from build123d import *

# Parameters (mm, degrees)
SKETCH_1_W          = 95
SKETCH_1_H          = 36
SKETCH_1_R          = 1.75
EXTRUDE_1_DEPTH     = 13
SKETCH_2_R          = 11
CUT_EXTRUDE_1_DEPTH = 96
SKETCH_4_R          = 3
SKETCH_4_R_2        = 1.25
CUT_EXTRUDE_2_DEPTH = 5


with BuildPart() as part:
    # Эскиз1 → Бобышка-Вытянуть1 (new body)
    with BuildSketch(Plane(origin=(0, 0, 0), x_dir=(1, 0, 0), z_dir=(0, 1, 0))):
        with Locations((47.5, 18)):
            Rectangle(SKETCH_1_W, SKETCH_1_H)
        with Locations((7.5, 32.5)):
            Circle(SKETCH_1_R, mode=Mode.SUBTRACT)
        with Locations((47.5, 32.5)):
            Circle(SKETCH_1_R, mode=Mode.SUBTRACT)
        with Locations((87.5, 32.5)):
            Circle(SKETCH_1_R, mode=Mode.SUBTRACT)
        with Locations((87.5, 3.5)):
            Circle(SKETCH_1_R, mode=Mode.SUBTRACT)
        with Locations((47.5, 3.5)):
            Circle(SKETCH_1_R, mode=Mode.SUBTRACT)
        with Locations((7.5, 3.5)):
            Circle(SKETCH_1_R, mode=Mode.SUBTRACT)
    extrude(amount=EXTRUDE_1_DEPTH)

    # Эскиз2 → Вырез-Вытянуть1 (cut, through all)
    with BuildSketch(Plane(origin=(95, 0, 0), x_dir=(0, 0, -1), z_dir=(1, 0, 0))):
        with Locations((18, 13)):
            Circle(SKETCH_2_R)
    extrude(amount=-CUT_EXTRUDE_1_DEPTH, mode=Mode.SUBTRACT)

    # Эскиз4 → Вырез-Вытянуть2 (cut)
    with BuildSketch(Plane(origin=(0, 13, 0), x_dir=(1, 0, 0), z_dir=(0, 1, 0))):
        with Locations((7.5, 32.5)):
            Circle(SKETCH_4_R)
        with Locations((47.5, 32.5)):
            Circle(SKETCH_4_R)
        with Locations((87.5, 32.5)):
            Circle(SKETCH_4_R)
        with Locations((87.5, 3.5)):
            Circle(SKETCH_4_R)
        with Locations((47.5, 3.5)):
            Circle(SKETCH_4_R)
        with Locations((7.5, 3.5)):
            Circle(SKETCH_4_R)
        with Locations((27.5, 34)):
            Circle(SKETCH_4_R_2)
        with Locations((67.5, 34)):
            Circle(SKETCH_4_R_2)
        with Locations((67.5, 2)):
            Circle(SKETCH_4_R_2)
        with Locations((27.5, 2)):
            Circle(SKETCH_4_R_2)
    extrude(amount=-CUT_EXTRUDE_2_DEPTH, mode=Mode.SUBTRACT)


solid = part.part
Design review of the part built by this model. Coordinates are the model's own, in mm. A direction names the side the tool comes from. Coordinates: 2 decimals unless noted, no trailing zeros. Order: outer loops, then holes, each group sorted by start corner. A loop starts at its lowest first (then second) coordinate and runs counter-clockwise, first axis right, second up.
Item 1: Take a section at A-A, the plane y = 4.75. Write out the cut boundary in (x, z), then the cut area to 3 significant figures.
Item 2: For line 1 (X direction, y = 2.5, z = -32.5); line 2 (X direction, y = 12, z = -32.5); line 3 (Z direction, x = 89, y = 4), list the stretches that pass through material, from the lowest coordinate up.
Item 3: Take a section at D-D, the plane x = 67.5. Write out the cut boundary in (y, z), then the cut area to 3 significant figures.
Item 4: Take a section at B-B, the plane x = 7.5. Write out the cut boundary in (y, z), then the cut area to 3 significant figures.
Item 5: The part is to be moulded in two halves that separate along Z. For faces 3 (the flat face through (47, 6, -36)), 4 (the flat face through (0, 1, -18)), 5 (the cylindrical face through (44.5, 10.5, -3.6)), say which applies: pulls with the +Z half, pulls with the -Z half, needs draft (parallel to the pull), parting line crosses it, or undercut.
Item 6: For pin 1 Ø0.8 at (x, z) = (28, -34.5) entering from +Y, flat-tipped, find the tip position at first contact; note if it passes through.
Item 7: For faces 1 (the cylindrical face through (89.169, 3.944, -4.026)), 2 (the cylindrical face through (10.36, 10.54, -33.4)), list the 3-axis set-ups (+Z, -Z, +X, -X, +Y, -Y) from which the entire face can be reached by the end or side of a thin tool; tool diameter is ignored.
Item 8: Take a section at C-C, the plane y = 9.75. Count the separate pieces of the cut face and the enclosed holes in it, then the cut area to 3 significant figures.
The answers:
1. outline: (0, -36) - (95, -36) - (95, -25.28) - (0, -25.28) - close; (0, -10.72) - (95, -10.72) - (95, 0) - (0, 0) - close; hole circle Ø3.5 at (7.5, -32.5); hole circle Ø3.5 at (7.5, -3.5); hole circle Ø3.5 at (47.5, -32.5); hole circle Ø3.5 at (47.5, -3.5); hole circle Ø3.5 at (87.5, -32.5); hole circle Ø3.5 at (87.5, -3.5)
1. area: 1,980 mm2
2. line 1: x = 0 to 5.75, 9.25 to 45.75, 49.25 to 85.75, 89.25 to 95
2. line 2: x = 0 to 4.5, 10.5 to 44.5, 50.5 to 84.5, 90.5 to 95
2. line 3: z = -36 to -33.4, -31.6 to -24.32, -11.68 to -4.4, -2.6 to 0
3. outline: (0, -36) - (13, -36) - (13, -35.25) - (8, -35.25) - (8, -32.75) - (13, -32.75) - (13, -29) arc R11 cw to (13, -7) - (13, -3.25) - (8, -3.25) - (8, -0.75) - (13, -0.75) - (13, 0) - (0, 0) - close
3. area: 253 mm2
4. outline: (0, -36) - (13, -36) - (13, -35.5) - (8, -35.5) - (8, -34.25) - (0, -34.25) - close; (0, -30.75) - (8, -30.75) - (8, -29.5) - (13, -29.5) - (13, -29) arc R11 cw to (13, -7) - (13, -6.5) - (8, -6.5) - (8, -5.25) - (0, -5.25) - close; (0, -1.75) - (8, -1.75) - (8, -0.5) - (13, -0.5) - (13, 0) - (0, 0) - close
4. area: 162 mm2
5. face 3: pulls with the -Z half
5. face 4: needs draft
5. face 5: undercut
6. pin 1: stops at y = 8
7. face 1: +Y, -Y
7. face 2: +Y
8. separate pieces: 2
8. enclosed holes: 10
8. area: 1,230 mm2
